from build123d import *

# Parameters (mm, degrees)
F0_R     = 6
F1_DEPTH = 10
F3_DEPTH = 3


with BuildPart() as f1:
    # F0 (on Top) → F1 (new body)
    with BuildSketch(Plane.XY):
        Polygon((10, 0), (0, 0), (-10, 0), (-20, 0), (-20, -10), (-30, -10), (-40, -10), (-50, -10), (-50, -20), (-60, -20), (-60, -30), (-60, -40), (-60, -50), (-50, -50), (-40, -50), (-40, -60), (-50, -60), (-50, -70), (-40, -70), (-40, -80), (-30, -80), (-20, -80), (-20, -70), (-30, -70), (-30, -60), (-20, -60), (-10, -60), (-10, -70), (0, -70), (10, -70), (10, -60), (20, -60), (30, -60), (30, -70), (20, -70), (20, -80), (30, -80), (40, -80), (40, -70), (50, -70), (50, -60), (40, -60), (40, -50), (50, -50), (60, -50), (60, -40), (60, -30), (60, -20), (50, -20), (50, -10), (40, -10), (30, -10), (20, -10), (20, 0), align=None)
        Polygon((-10, -45), (0, -45), (10, -45), (10, -55), (0, -55), (-10, -55), align=None, mode=Mode.SUBTRACT)
        Polygon((-30, -30), (-30, -20), (-20, -20), (-10, -20), (-10, -30), (-20, -30), align=None, mode=Mode.SUBTRACT)
        Polygon((10, -20), (20, -20), (30, -20), (30, -30), (20, -30), (10, -30), align=None, mode=Mode.SUBTRACT)
        with Locations((0, -12)):
            Circle(F0_R, mode=Mode.SUBTRACT)
        with Locations((0, -12)):
            Circle(F0_R)
    extrude(amount=F1_DEPTH)

    # F2 (on Right) → F3 (cut, symmetric)
    with BuildSketch(Plane.YZ):
        Polygon((-16, 5), (-16, 0), (-10, 0), (-7.1132486541, 5), align=None)
    extrude(amount=F3_DEPTH, both=True, mode=Mode.SUBTRACT)


solid = f1.part
Could you check a few things on this model? Use its own coordinates, in mm. A direction names the side the tool comes from. Give positions to 0.01 mm unless a question says otherwise; leave off trailing zeros. Write each loop counter-clockwise with the first axis right and the second up, starting at its lowest first coordinate (ties: lowest second). Pieces come first, ordered by that corner, then holes. Notation, with made-up numbers: (-6.5, 62.25) -> (47.5, 62.25) arc R28 ccw to (47.5, 94.25) -> close; hole circle Ø8 at (-32, 47.5). An arc over 180 degrees is marked (long way). Answer as a JSON object with one key per item and string values.
Q1. Suppose I cut it at B-B on y = -25. Write out the boundary of the cut face in (x, z).
Taken from the geometry:
{"outline": "(-60, 0) -> (-30, 0) -> (-30, 10) -> (-60, 10) -> close; (-10, 0) -> (10, 0) -> (10, 10) -> (-10, 10) -> close; (30, 0) -> (60, 0) -> (60, 10) -> (30, 10) -> close"}
Q2. Which directions (+Z, -Z, +X, -X, +Y, -Y) give clear straight access to the entire face, cutting with the end or side of a thin tool? Please do faces 1 (the flat face through (0, -11, 5)), 2 (the flat face through (50, -65, 5)), 3 (the flat face through (0, -70, 5)), 4 (the flat face through (30, -25, 5)), 5 (the flat face through (55, -20, 5)).
Taken from the geometry:
{"face 1": "none", "face 2": "+Z, -Z, +X, -Y", "face 3": "+Z, -Z, -Y", "face 4": "+Z, -Z", "face 5": "+Z, -Z, +X, +Y"}
Q3. We'd pull the mould along X, two halves only. Please class faces 6 (the flat face through (-10, -25, 5)), 7 (the flat face through (-20, -5, 5)), 8 (the flat face through (-50, -50, 5)), 9 (the flat face through (20, -5, 5)): released by +X, released by -X, zero draft, split by the parting line, or undercut.
Taken from the geometry:
{"face 6": "undercut", "face 7": "released by -X", "face 8": "zero draft", "face 9": "released by +X"}
Q4. Will these pins go through, and if not, where does the flat tip stop? pin 1 Ø5 at (y, z) = (-16, 4.5) entering from +X; pin 2 Ø3 at (y, z) = (-55.5, 3.5) entering from -X; pin 3 Ø3 at (x, z) = (25, 3) entering from +Y.
Taken from the geometry:
{"pin 1": "stops at x = 50", "pin 2": "stops at x = -40", "pin 3": "stops at y = -10"}
Q5. Please list where these lines run through material, in increasing order: L1, parallel to Y at x = -28.5, z = 4.25; L2, parallel to X at y = -26, z = 8.5; L3, parallel to X at y = -65, z = 8.
Taken from the geometry:
{"L1": "y = -80 to -70, -60 to -30, -20 to -10", "L2": "x = -60 to -30, -10 to 10, 30 to 60", "L3": "x = -50 to -30, -10 to 10, 30 to 50"}
Q6. Suppose I cut it at A-A on x = -1. Write out the boundary of the cut face in (y, z).
Taken from the geometry:
{"outline": "(-70, 0) -> (-55, 0) -> (-55, 10) -> (-70, 10) -> close; (-45, 0) -> (-16, 0) -> (-16, 5) -> (-7.11, 5) -> (-10, 0) -> (0, 0) -> (0, 10) -> (-45, 10) -> close"}
Q7. Suppose I cut it at D-D on z = 3.5. Count the separate pieces of the cut face and the enclosed holes in it, then the cut area to 3 significant figures.
Taken from the geometry:
{"separate pieces": "1", "enclosed holes": "4", "area": "6,150 mm²"}
Q8. Suppose I cut it at C-C on x = -23. Write out the boundary of the cut face in (y, z), then the cut area to 3 significant figures.
Taken from the geometry:
{"outline": "(-80, 0) -> (-70, 0) -> (-70, 10) -> (-80, 10) -> close; (-60, 0) -> (-30, 0) -> (-30, 10) -> (-60, 10) -> close; (-20, 0) -> (-10, 0) -> (-10, 10) -> (-20, 10) -> close", "area": "500 mm²"}
